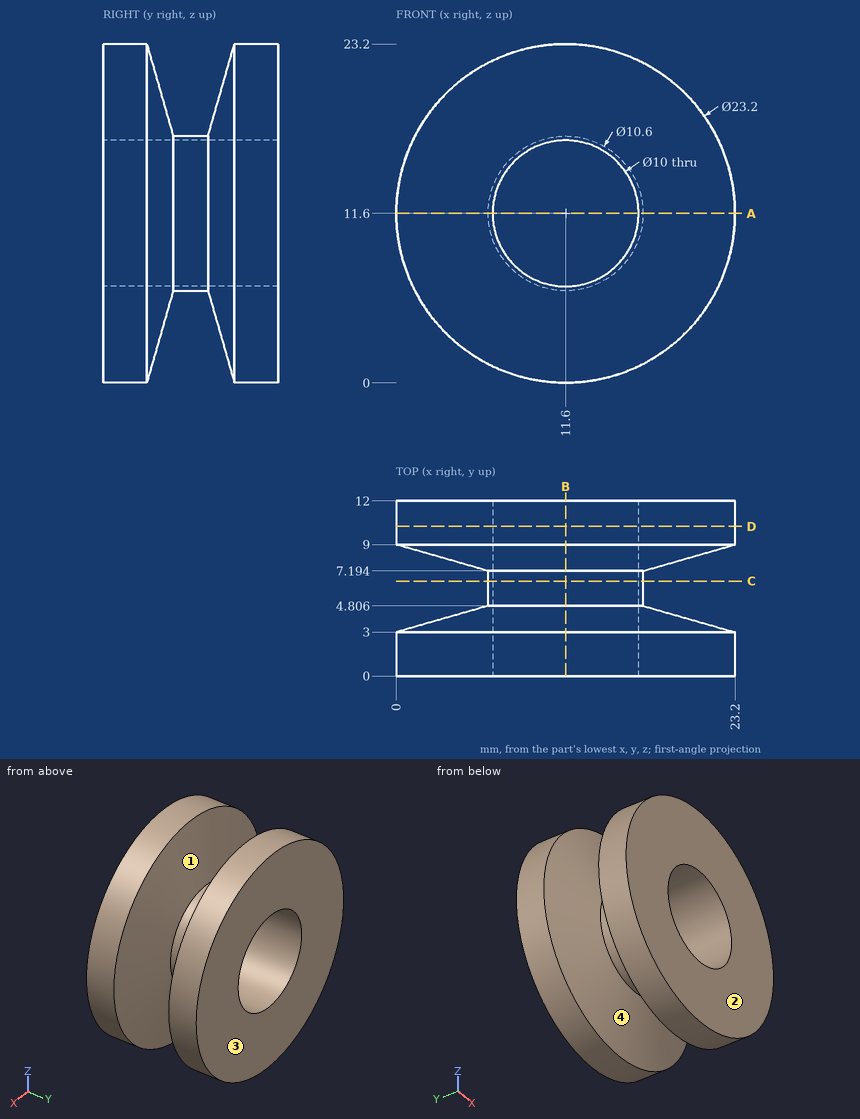
Design review of the part shown in the three views and the two pictorial views. Dimensions are in mm from the part's minimum x, y and z. Round coordinates to 2 decimals unless told otherwise and drop trailing zeros. Order: outer loops, then holes, each group sorted by start corner. A loop starts at its lowest first (then second) coordinate and runs counter-clockwise, first axis right, second up. Notation, with made-up numbers: (49, 80.25) -> (77, 80.25) arc R11 cw to (77, 92.25) -> close; hole circle Ø10 at (74.5, 13). An arc over 180 degrees is marked (long way). Write item = value, one per line. Start each with the question number.
1) Insertion check: pin 1 (2 mm diameter, centred on y = 3.5, z = 17, fed in from +X). The pin has a flat end and moves straight along its axis. Give the tip position at first contact, or say it passes through.
2) The part is to be moulded in two halves that separate along Y. For the marked faces 1, 2, 3 and 4, say which applies: +Y half, -Y half, draft (parallel to the pull), parting line (faces both ways), or undercut.
3) Take a section at D-D on y = 10.25. State the section outline as (x, z) points.
4) Take a section at C-C on y = 6.5. State the section outline as (x, z) points.
5) To check wall thickness, follow line 1 (X direction, y = 2.5, z = 11.5); line 2 (Y direction, x = 2, z = 9.5); line 3 (Y direction, x = 20.25, z = 7.75). State the ranges of each line that lie inside material, in increasing order. Write a range as from..to.
6) Take a section at A-A on z = 11.6. State the section outline as (x, y) points.
7) Take a section at B-B on x = 11.6. State the section outline as (y, z) points.
Verdict:
q1.pin_1 = 22.28
q2.face_1 = undercut
q2.face_2 = -Y half
q2.face_3 = +Y half
q2.face_4 = undercut
q3.outline = circle Ø23.2 at (11.6, 11.6); hole circle Ø10 at (11.6, 11.6)
q4.outline = circle Ø10.6 at (11.6, 11.6); hole circle Ø10 at (11.6, 11.6)
q5.line_1 = 0..6.6, 16.6..23.2
q5.line_2 = 0..3.51, 8.49..12
q5.line_3 = 0..3.61, 8.39..12
q6.outline = (0, 0) -> (6.6, 0) -> (6.6, 12) -> (0, 12) -> (0, 9) -> (6.3, 7.19) -> (6.3, 4.81) -> (0, 3) -> close; (16.6, 0) -> (23.2, 0) -> (23.2, 3) -> (16.9, 4.81) -> (16.9, 7.19) -> (23.2, 9) -> (23.2, 12) -> (16.6, 12) -> close
q7.outline = (0, 0) -> (3, 0) -> (4.81, 6.3) -> (7.19, 6.3) -> (9, 0) -> (12, 0) -> (12, 6.6) -> (0, 6.6) -> close; (0, 16.6) -> (12, 16.6) -> (12, 23.2) -> (9, 23.2) -> (7.19, 16.9) -> (4.81, 16.9) -> (3, 23.2) -> (0, 23.2) -> close
